from build123d import *

# Parameters (mm, degrees)
SKETCH_W     = 20
SKETCH_H     = 20
SKETCH_W_2   = 14
SKETCH_H_2   = 14
PAD_DEPTH    = 5
SKETCH001_W  = 16
SKETCH001_H  = 5
POCKET_DEPTH = 3.5


with BuildPart() as part:
    # Sketch → Pad (new body)
    with BuildSketch(Plane.XY):
        Rectangle(SKETCH_W, SKETCH_H)
        Rectangle(SKETCH_W_2, SKETCH_H_2, mode=Mode.SUBTRACT)
    extrude(amount=PAD_DEPTH)

    # Sketch001 → Pocket (cut)
    with BuildSketch(Plane.XY):
        Rectangle(SKETCH001_W, SKETCH001_H)
    extrude(amount=POCKET_DEPTH, mode=Mode.SUBTRACT)


solid = part.part
Source: CAD feature listing. Evaluate the final solid. Frame: model axes, mm. A direction names the side the tool comes from. Give positions to 0.01 mm unless a question says otherwise; leave off trailing zeros. Write each loop counter-clockwise with the first axis right and the second up, starting at its lowest first coordinate (ties: lowest second). Pieces come first, ordered by that corner, then holes. Notation, with made-up numbers: M 62,12 L 77,12 A24 ccw 77,26 Z; hole C 51,11 d11. An arc over 180 degrees is marked long. Answer as a JSON object with one key per item and string values.
Q1. Cut plane B-B, the plane z = 4.6. Return the cut outline in (x, y), then the cut area to 3 significant figures.
Geometry check:
{"outline": "M -10,-10 L 10,-10 L 10,10 L -10,10 Z; hole M -7,-7 L 7,-7 L 7,7 L -7,7 Z", "area": "204 mm^2"}
Q2. Cut plane D-D, the plane y = -0.5. Return the cut outline in (x, z).
Geometry check:
{"outline": "M -10,0 L -8,0 L -8,3.5 L -7,3.5 L -7,5 L -10,5 Z; M 7,3.5 L 8,3.5 L 8,0 L 10,0 L 10,5 L 7,5 Z"}
Q3. Cut plane A-A, the plane y = -2.75. Return the cut outline in (x, z), then the cut area to 3 significant figures.
Geometry check:
{"outline": "M -10,0 L -7,0 L -7,5 L -10,5 Z; M 7,0 L 10,0 L 10,5 L 7,5 Z", "area": "30.0 mm^2"}
Q4. Ray query, line 1 along X through (y, z) = (4.5, 1.95); line 2 along Y through (x, z) = (7.5, 1.1). Return the intervals inside material, ascending.
Geometry check:
{"line 1": "x = -10 to -7, 7 to 10", "line 2": "y = -10 to -2.5, 2.5 to 10"}
Q5. Access query for faces 5 (the face through (0, -7, 2)), 6 (the face through (7.5, -2.5, 1.7)), 7 (the face through (-9, 0, 0)). Directions: +Z, -Z, +X, -X, +Y, -Y. A direction counts if a zero-diameter tool reaches every point of the face in a straight line with its end or side. Return the directions, or none.
Geometry check:
{"face 5": "+Z, -Z", "face 6": "-Z", "face 7": "-Z, +X, -X, +Y, -Y"}
Q6. Contact query for a flat-ended pin moving along its axis: P1, Ø0.5, axis at x = -7.5, y = 0.5, coming from the -Z side. Output: stop coordinate, or through.
Geometry check:
{"P1": "stops at z = 3.5"}
Q7. Mould query, pull axis X, two halves, no side actions, for faces 1 (the face through (-10, 0, 2)), 2 (the face through (10, 0, 2)), 3 (the face through (-7.5, -2.5, 1.7)), 4 (the face through (0, 10, 2)). Classes: +X half, -X half, draft (parallel to the pull), parting line (faces both ways), or undercut.
Geometry check:
{"face 1": "-X half", "face 2": "+X half", "face 3": "undercut", "face 4": "draft"}
